from build123d import *

# Parameters (mm, degrees)
BOSS_EXTRUDE1_DEPTH = 3
SKETCH2_R           = 1
SKETCH2_W           = 7
SKETCH2_H           = 23.92041254
SKETCH2_H_2         = 5
BOSS_EXTRUDE4_DEPTH = 29
BOSS_EXTRUDE5_DEPTH = 7
SKETCH2_4_R         = 1
CUT_EXTRUDE1_DEPTH  = 29


with BuildPart() as part:
    # Sketch1 → Boss-Extrude1 (new body)
    with BuildSketch(Plane(origin=(0, 0, 0), x_dir=(1, 0, 0), z_dir=(0, 1, 0))):
        Polygon((86.602540378, 0), (43.301270189, 75), (-43.301270189, 75), (-86.602540378, 0), (-43.301270189, -75), (43.301270189, -75), align=None)
    extrude(amount=BOSS_EXTRUDE1_DEPTH)

    # Sketch2 → Boss-Extrude4 (add)
    # profile 1 of 5: a face of its own
    with BuildSketch(Plane(origin=(0, 3, 0), x_dir=(1, 0, 0), z_dir=(0, 1, 0))):
        with Locations(Location((-14.1, -4.8, 0), (0, 0, 90))):
            Circle(SKETCH2_R)
    # profile 2 of 5: a face of its own
    with BuildSketch(Plane(origin=(0, 3, 0), x_dir=(1, 0, 0), z_dir=(0, 1, 0))):
        with Locations(Location((-14.1, 4.8, 0), (0, 0, 90))):
            Circle(SKETCH2_R)
    # profile 3 of 5: a face of its own
    with BuildSketch(Plane(origin=(0, 3, 0), x_dir=(1, 0, 0), z_dir=(0, 1, 0))):
        with Locations((32.9, 0)):
            Rectangle(SKETCH2_W, SKETCH2_H)
        with Locations(Location((33.9, -4.8, 0), (0, 0, 90))):
            Circle(SKETCH2_R, mode=Mode.SUBTRACT)
        with Locations(Location((33.9, 4.8, 0), (0, 0, 90))):
            Circle(SKETCH2_R, mode=Mode.SUBTRACT)
    # profile 4 of 5: a face of its own
    with BuildSketch(Plane(origin=(0, 3, 0), x_dir=(1, 0, 0), z_dir=(0, 1, 0))):
        with Locations((-13.1, 9.46020627)):
            Rectangle(SKETCH2_W, SKETCH2_H_2)
    # profile 5 of 5: a face of its own
    with BuildSketch(Plane(origin=(0, 3, 0), x_dir=(1, 0, 0), z_dir=(0, 1, 0))):
        with Locations((-13.1, -9.46020627)):
            Rectangle(SKETCH2_W, SKETCH2_H_2)
    extrude(amount=BOSS_EXTRUDE4_DEPTH)

    # Sketch4 → Boss-Extrude5 (add)
    with BuildSketch(Plane.ZY.offset(16.6)):
        Polygon((-6.96020627, 12), (0, 22), (6.96020627, 12), (6.96020627, 32), (-6.96020627, 32), align=None)
    extrude(amount=-BOSS_EXTRUDE5_DEPTH)

    # Sketch2<4> → Cut-Extrude1 (cut)
    with BuildSketch(Plane(origin=(0, 3, 0), x_dir=(1, 0, 0), z_dir=(0, 1, 0))):
        with Locations(Location((-14.1, -4.8, 0), (0, 0, 90))):
            Circle(SKETCH2_4_R)
        with Locations(Location((-14.1, 4.8, 0), (0, 0, 90))):
            Circle(SKETCH2_4_R)
    extrude(amount=CUT_EXTRUDE1_DEPTH, mode=Mode.SUBTRACT)


solid = part.part
Work out the finished part from the listing and answer in its coordinate system (mm). A direction names the side the tool comes from. Give positions to 0.01 mm unless a question says otherwise; leave off trailing zeros. Order: outer loops, then holes, each group sorted by start corner. A loop starts at its lowest first (then second) coordinate and runs counter-clockwise, first axis right, second up. Notation, with made-up numbers: M 58.25,23.25 L 105.25,23.25 A24 ccw 105.25,34.25 Z; hole C 40.25,10.5 d9. An arc over 180 degrees is marked long. Return JSON: item names as keys, results as strings.
Q1. Find section B-B, the plane y = 29. Write down the section's boundary in (x, z).
Answer below:
{"outline": "M -16.6,-11.96 L -9.6,-11.96 L -9.6,11.96 L -16.6,11.96 Z; M 29.4,-11.96 L 36.4,-11.96 L 36.4,11.96 L 29.4,11.96 Z; hole C -14.1,-4.8 d2; hole C -14.1,4.8 d2; hole C 33.9,-4.8 d2; hole C 33.9,4.8 d2"}
Q2. Which of the six approach directions +Z, -Z, +X, -X, +Y, -Y give full straight-line access (tool end or side, diameter ignored) to faces 4 (the face through (-16.6, 21, -3)), 5 (the face through (-13, 17, 11.96)), 6 (the face through (-13, 7, -6.96))?
Answer below:
{"face 4": "+Z, -Z, -X, +Y", "face 5": "+Z, +X, -X, +Y", "face 6": "-X"}
Q3. Find section D-D, the plane x = 0.5. Write down the section's boundary in (y, z).
Answer below:
{"outline": "M 0,-75 L 3,-75 L 3,75 L 0,75 Z"}
Q4. The mould has two halves that part along Z. Classify faces 1 (the face through (-9.6, 21, -3)), 2 (the face through (-13.15, 17.07, 3.43)), 3 (the face through (-65.255, 1.479, 36.975)): pulls with the +Z half, pulls with the -Z half, needs draft (parallel to the pull), parting line crosses it, or undercut.
Answer below:
{"face 1": "needs draft", "face 2": "undercut", "face 3": "pulls with the +Z half"}
Q5. Each of these flat-tipped pins is pushed along its axis until it touches: pin 1 (3.5 mm diameter, centred on x = -15, y = 15, fed in from +Z); pin 2 (2 mm diameter, centred on x = 34.5, y = 16, fed in from -Z); pin 3 (12 mm diameter, centred on y = 14.5, z = 4, fed in from +X). Where does it stop, or does it pass through?
Answer below:
{"pin 1": "stops at z = 11.96", "pin 2": "stops at z = -11.96", "pin 3": "stops at x = 36.4"}
Q6. Find section A-A, the plane y = 9.5. Write down the section's boundary in (x, z), and give its area (3 significant figures).
Answer below:
{"outline": "M -16.6,-11.96 L -9.6,-11.96 L -9.6,-6.96 L -16.6,-6.96 Z; M -16.6,6.96 L -9.6,6.96 L -9.6,11.96 L -16.6,11.96 Z; M 29.4,-11.96 L 36.4,-11.96 L 36.4,11.96 L 29.4,11.96 Z; hole C 33.9,-4.8 d2; hole C 33.9,4.8 d2", "area": "231 mm^2"}
Q7. Find section C-C, the plane y = 20. Write down the section's boundary in (x, z), and give its area (3 significant figures).
Answer below:
{"outline": "M -16.6,-11.96 L -9.6,-11.96 L -9.6,-1.39 L -16.6,-1.39 Z; M -16.6,1.39 L -9.6,1.39 L -9.6,11.96 L -16.6,11.96 Z; M 29.4,-11.96 L 36.4,-11.96 L 36.4,11.96 L 29.4,11.96 Z; hole C -14.1,-4.8 d2; hole C -14.1,4.8 d2; hole C 33.9,-4.8 d2; hole C 33.9,4.8 d2", "area": "303 mm^2"}
Q8. Find the intervals of material crossed by line 1 along X through (y, z) = (17.5, 4.5); line 2 along Z through (x, y) = (33.9, 25); line 3 along X through (y, z) = (18, -5.5), in increasing order. Write a range as [from, to].
Answer below:
{"line 1": "x = [-16.6, -15.05], [-13.15, -9.6], [29.4, 32.95], [34.85, 36.4]", "line 2": "z = [-11.96, -5.8], [-3.8, 3.8], [5.8, 11.96]", "line 3": "x = [-16.6, -14.81], [-13.39, -9.6], [29.4, 33.19], [34.61, 36.4]"}
